Check sheet for the drawn part. Datum: minimum x, y, z corner. Units: mm. A direction names the side the tool comes from. Give positions to 0.01 mm unless a question says otherwise; leave off trailing zeros. Write each loop counter-clockwise with the first axis right and the second up, starting at its lowest first coordinate (ties: lowest second). Pieces come first, ordered by that corner, then holes. Notation, with made-up numbers: (34, 88) - (62, 88) arc R30 ccw to (62, 120) - close; hole circle Ø11 at (-23, 89.25). An arc over 180 degrees is marked (long way). Answer as a JSON object with one key per item and string values. Group by question number.
Item 1: Scan lines: line 1 along X through (y, z) = (4.75, 9.5); line 2 along Y through (x, z) = (36, 23.5); line 3 along X through (y, z) = (1.5, 23). Record each from-to range of solid material in increasing order. Write a range as [from, to].
Item 2: Sectioned sample at C-C, the plane z = 41. Record the boundary of the cut face in (x, y).
Item 3: Go/stop test with flat-tipped pins: pin 1 (1.5 mm diameter, centred on x = 34, z = 4, fed in from +Y); pin 2 (3.5 mm diameter, centred on x = 9, z = 2, fed in from -Y); pin 3 (2.5 mm diameter, centred on x = 13, y = 7, fed in from +Z). Record where each tip stops, or that it passes through.
Item 4: Sectioned sample at B-B, the plane x = 31. Record the boundary of the cut face in (y, z), and give its area (3 significant figures).
Item 5: Sectioned sample at A-A, the plane y = 4.5. Record the boundary of the cut face in (x, z).
Item 6: Draft check along Z on the marked faces 4, 5, 6 and 7. Enter one of: +Z half, -Z half, draft (parallel to the pull), parting line (faces both ways), or undercut.
Item 7: Tool access check on the marked faces 1, 2 and 3. Record the directions out of +Z, -Z, +X, -X, +Y, -Y that give a thin tool (end or side, any length) a straight path to the whole face; none if there is none.
Item 8: Sectioned sample at D-D, the plane y = 0.5. Record the boundary of the cut face in (x, z), and give its area (3 significant figures).
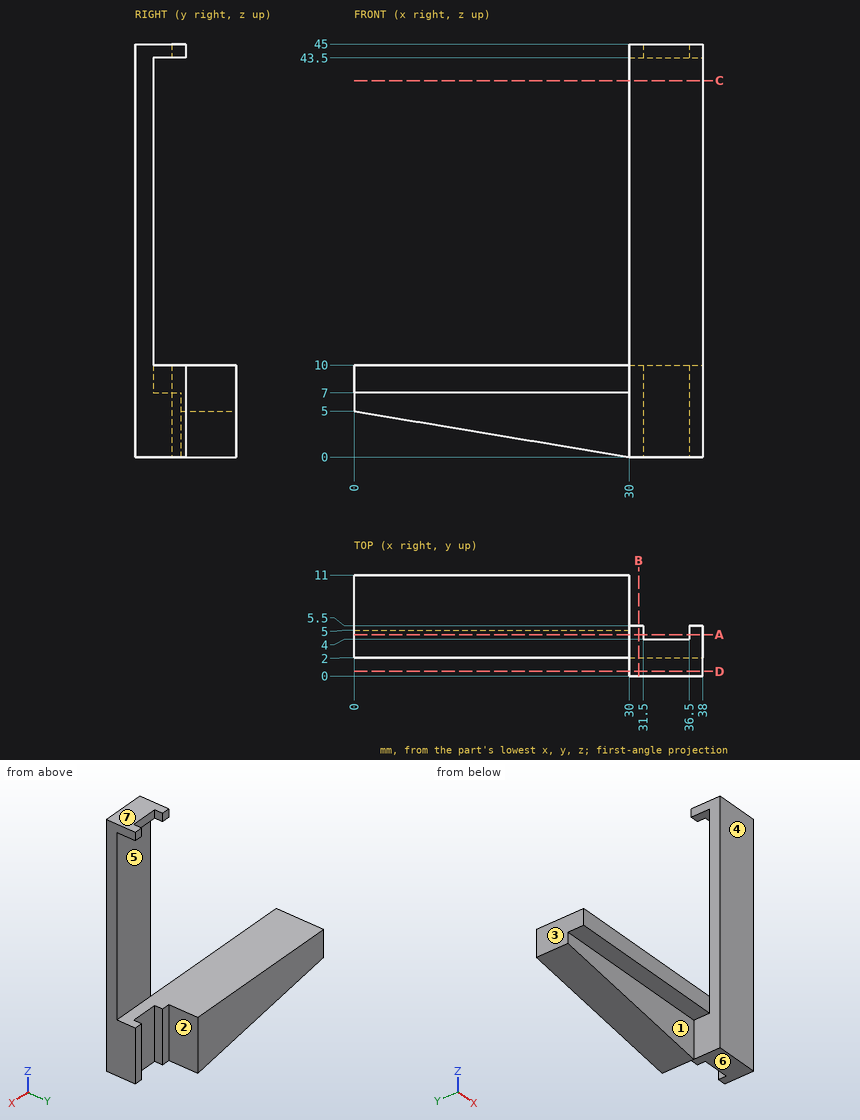
Geometry check:
{
 "1": {"line 1": "[0, 31.5], [36.5, 38]", "line 2": "[0, 2]", "line 3": "[30, 38]"},
 "2": {"outline": "(30, 0) - (38, 0) - (38, 2) - (30, 2) - close"},
 "3": {"pin 1": "y = 4", "pin 2": "y = 5", "pin 3": "z = 10"},
 "4": {"outline": "(0, 0) - (5.5, 0) - (5.5, 10) - (2, 10) - (2, 43.5) - (5.5, 43.5) - (5.5, 45) - (0, 45) - close", "area": "130 mm^2"},
 "5": {"outline": "(0, 7) - (30, 7) - (30, 0) - (31.5, 0) - (31.5, 10) - (0, 10) - close; (30, 43.5) - (31.5, 43.5) - (31.5, 45) - (30, 45) - close; (36.5, 0) - (38, 0) - (38, 10) - (36.5, 10) - close; (36.5, 43.5) - (38, 43.5) - (38, 45) - (36.5, 45) - close"},
 "6": {"face 4": "draft", "face 5": "undercut", "face 6": "-Z half", "face 7": "+Z half"},
 "7": {"face 1": "-Z, -X, -Y", "face 2": "+Z, -Z, +X, +Y", "face 3": "+Z, -Z, -X, +Y, -Y"},
 "8": {"outline": "(30, 0) - (38, 0) - (38, 45) - (30, 45) - close", "area": "360 mm^2"}
}
